Input: part model. Units: mm. Frame: model coordinates. Face numbers are marked on the shaded views. Give positions to 0.01 mm unless a question says otherwise; leave off trailing zeros. Order: outer loops, then holes, each group sorted by start corner. A loop starts at its lowest first (then second) coordinate and runs counter-clockwise, first axis right, second up.
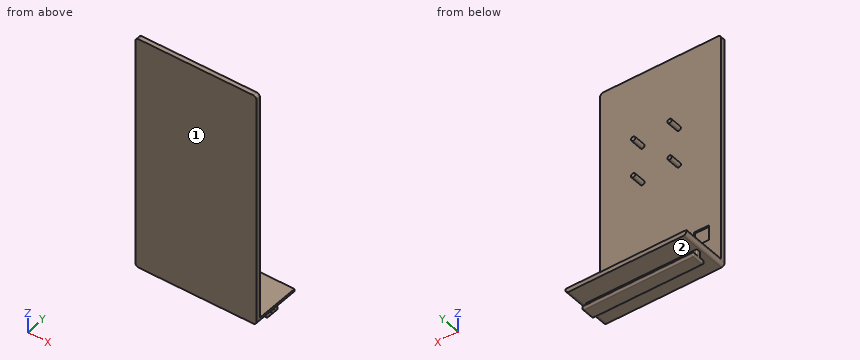
Autodesk Inventor part; units mm, degrees
ref_plane "YZ Plane" through (0, 0, 0) normal (1, 0, 0) x (0, 1, 0)
ref_plane "XZ Plane" through (0, 0, 0) normal (0, 1, 0) x (-1, 0, 0)
ref_plane "XY Plane" through (0, 0, 0) normal (0, 0, 1) x (1, 0, 0)
sketch "Sketch1" plane through (0, 0, 0) normal (0, 1, 0) x (-1, 0, 0)
  line L0 (-40, -78) -> (40, -78)
  line L1 (40, -78) -> (40, 78)
  line L2 (40, 78) -> (-40, 78)
  line L3 (-40, 78) -> (-40, -78)
  line L4 (-40, -78) -> (40, 78) construction
  line L5 (40, -78) -> (-40, 78) construction
  point P0 (0, 0)
  dimension "d0" = 80
  dimension "d1" = 156
extrude "Extrusion1" add sketch "Sketch1" along normal blind 3
sketch "Sketch2" plane through (0, 3, 0) normal (0, 1, 0) x (1, 0, 0)
  line L0 (-40, 78) -> (-40, -78)
  line L1 (-40, -78) -> (40, -78)
  line L2 (40, -78) -> (40, 78)
  line L3 (40, 78) -> (-40, 78)
  line L4 (40, 78) -> (-40, 78)
  line L5 (-40, 78) -> (-40, -78)
  line L6 (-40, -78) -> (40, -78)
  line L7 (40, -78) -> (40, 78)
  line L8 (40, 78) -> (-40, -78) construction
  line L9 (-40, 78) -> (40, -78) construction
  line L10 (37, 75) -> (-37, 75)
  line L11 (-37, 75) -> (-37, -75)
  line L12 (-37, -75) -> (37, -75)
  line L13 (37, -75) -> (37, 75)
  line L14 (37, 75) -> (-37, -75) construction
  line L15 (-37, 75) -> (37, -75) construction
  point P0 (0, 0)
  dimension "d4" = 0
  dimension "d5" = 0
  dimension "d6" = 3
  dimension "d7" = 3
extrude "Extrusion2" add sketch "Sketch2" along normal blind 30
fillet "Fillet1" radius 2 4 edges at (40, 16.5, 78) (40, 16.5, -78) (-40, 16.5, 78) (-40, 16.5, -78)
sketch "Sketch13" plane through (23.2, 5, -78) normal (0, 0, -1) x (-1, 0, 0)
  line L0 (-13.8, 18) -> (60.2, 18)
  line L1 (60.2, 18) -> (60.2, 8.4)
  line L2 (60.2, 8.4) -> (-13.8, 8.4)
  line L3 (-13.8, 8.4) -> (-13.8, 18)
  line L4 (63.2, -5) -> (63.2, 28)
  line L5 (-16.8, 28) -> (-16.8, -5)
  line L6 (-14.8, -5) -> (61.2, -5)
  point P0 (23.2, -5)
  point P1 (51.4, 0)
  point P2 (-5, 0)
  point P3 (-16.8, -5)
  point P4 (63.2, 11.5)
  point P5 (60.2, 13.2)
  dimension "d131" = 9.6
  dimension "d146" = 3
  dimension "d147" = 3
  dimension "d156" = 23
extrude "Extrusion13" add sketch "Sketch13" along normal blind 6
sketch "Sketch14" plane through (-37, 13.4, -78) normal (-1, 0, 0) x (0, 0, 1)
  line L0 (0, 9.6) -> (0, 0)
  line L1 (0, 9.6) -> (-6, 9.6)
  line L2 (-6, 0) -> (-6, 9.6)
  line L3 (0, 0) -> (-6, 0)
  line L4 (0, 9.6) -> (-3.4, 9.6)
  line L5 (-3.4, 9.6) -> (-3.4, 6.6)
  line L6 (-3.4, 6.6) -> (0, 6.6)
  line L7 (0, 6.6) -> (0, 9.6)
  line L8 (0, 0) -> (-3.4, 0)
  line L9 (-3.4, 0) -> (-3.4, 3)
  line L10 (-3.4, 3) -> (0, 3)
  line L11 (0, 3) -> (0, 0)
  point P0 (78, -13.4)
  point P1 (0, 6.6)
  dimension "d137" = 3.4
  dimension "d138" = 3
  dimension "d139" = 3.4
  dimension "d140" = 3
extrude "Extrusion14" cut sketch "Sketch14" against normal up to surface (74 mm away) contours L0 L6 L5 L1 | L0 L3 L9 L10
fillet "Fillet5" radius 1 18 edges at (0, 23, -84) (0, 23, -81.4) (0, 13.4, -84) (0, 13.4, -81.4) (-37, 16.4, -79.7) (-37, 20, -79.7) (37, 16.4, -79.7) (37, 20, -79.7) (-37, 18.2, -84) (-37, 21.5, -81.4) (-37, 14.9, -81.4) (-37, 23, -82.7) (-37, 13.4, -82.7) (37, 23, -82.7) (37, 13.4, -82.7) (37, 14.9, -81.4) (37, 18.2, -84) (37, 21.5, -81.4)
sketch "Sketch16" plane through (0, 33, 0) normal (0, 1, 0) x (1, 0, 0)
  arc A0 (-38, 78) -> (-40, 76) centre (-38, 76) ccw
  line L0 (-40, 76) -> (-40, -76)
  arc A1 (-40, -76) -> (-38, -78) centre (-38, -76) ccw
  line L1 (-38, -78) -> (38, -78)
  arc A2 (38, -78) -> (40, -76) centre (38, -76) ccw
  line L2 (40, -76) -> (40, 76)
  arc A3 (40, 76) -> (38, 78) centre (38, 76) ccw
  line L3 (38, 78) -> (-38, 78)
  line L4 (37, 75) -> (37, -75)
  line L5 (37, -75) -> (-37, -75)
  line L6 (-37, -75) -> (-37, 75)
  line L7 (-37, 75) -> (37, 75)
  line L8 (-37, 75) -> (-40, 75)
  line L9 (37, 75) -> (40, 75)
  circle A4 centre (38, 76) radius 2
  circle A5 centre (-38, 76) radius 2
  point P0 (0, 0)
  point P1 (-39.7321, 75)
  point P2 (40, 76)
  point P3 (39.7321, 75)
  dimension "d180" = 4
  dimension "d181" = 4
extrude "Extrusion16" cut sketch "Sketch16" against normal blind 30 contours L8 A5 L6 L5 L4 A4 L9 L2 A2 L1 A1 L0 | L8 L6 A5 | A4 L4 L9
sketch "Sketch18" plane through (0, 3, 0) normal (0, 1, 0) x (1, 0, 0)
  line L0 (40, 75) -> (-40, 75)
  line L1 (38, -78) -> (-38, -78)
  line L2 (40, 75) -> (40, -76)
  line L3 (32, 58) -> (22, 58)
  line L4 (22, 58) -> (22, 48)
  line L5 (22, 48) -> (32, 48)
  line L6 (32, 48) -> (32, 58)
  line L7 (-22, 48) -> (-32, 48)
  line L8 (-32, 48) -> (-32, 58)
  line L9 (-32, 58) -> (-22, 58)
  line L10 (-22, 58) -> (-22, 48)
  line L11 (38, 78) -> (-38, 78)
  line L12 (-40, -76) -> (-40, 75)
  arc A0 (-40, -76) -> (-38, -78) centre (-38, -76) ccw
  arc A1 (38, -78) -> (40, -76) centre (38, -76) ccw
  dimension "d182" = 10
  dimension "d183" = 10
  dimension "d184" = 8
  dimension "d185" = 10
  dimension "d186" = 10
  dimension "d188" = 20
  dimension "d189" = 20
extrude "Extrusion18" cut sketch "Sketch18" against normal blind 1 contours L6 L5 L4 L3 | L7 L8 L9 L10
sketch "Sketch19" plane through (0, 3, 0) normal (0, 1, 0) x (1, 0, 0)
  line L0 (40, 75) -> (40, -76)
  line L1 (38, -78) -> (-38, -78)
  line L2 (-40, -76) -> (-40, 76)
  circle A0 centre (-12.05, -3) radius 1.45
  circle A1 centre (-12.05, -28) radius 1.45
  circle A2 centre (12.05, -3) radius 1.45
  circle A3 centre (12.05, -28) radius 1.45
  line L3 (-5, -54) -> (5, -54)
  line L4 (32, 58) -> (32, 48)
  line L5 (-32, 48) -> (-32, 58)
  point P0 (40, 76)
  point P1 (0, -54)
  point P2 (0, -54)
  point P3 (32, 53)
  point P4 (-32, 53)
  dimension "d215" = 2.9
  dimension "d216" = 2.9
  dimension "d217" = 2.9
  dimension "d218" = 2.9
  dimension "d219" = 25
  dimension "d220" = 25
  dimension "d221" = 24.1
  dimension "d222" = 12.05
  dimension "d223" = 12.05
  dimension "d224" = 56
  dimension "d225" = 56
extrude "Extrusion19" add sketch "Sketch19" along normal blind 8
properties part number "module_command" material "PC/ABS Plastic"
1) Cut plane A-A (y = 5). Return the cut outline in (x, z).
2) Line query: probe 1 along Y at (x, z) = (13.5, 42.5); probe 2 along Z at (x, y) = (10.5, 9); probe 3 along Y at (x, z) = (31.5, -50). Output: solid intervals per line, ascending.
3) Cut plane C-C (z = 9.5). Return the cut outline in (x, y), then the cut area to 3 significant figures.
4) Cut plane B-B (x = -19). Return the cut outline in (y, z), then the cut area to 3 significant figures.
5) First-contact query: P1, Ø8, axis at x = -4.5, z = -51, coming from the +Y side; P2, Ø8, axis at y = 10, z = 5.5, coming from the -X side; P3, Ø8, axis at x = -17.5, y = 23, coming from the +Z side. Flat tips, straight axial feed; report the tip coordinate or a pass-through.
6) Pull-direction query (Z, two-part tool) for the marked faces 1 and 2; classes: pulls with the +Z half, pulls with the -Z half, needs draft (parallel to the pull), parting line crosses it, or undercut.
Geometry says:
1. outline: (-40, -76) arc R2 ccw to (-38, -78) - (38, -78) arc R2 ccw to (40, -76) - (40, -75) - (-40, -75) - close; circle Ø2.9 at (-12.05, 3); circle Ø2.9 at (-12.05, 28); circle Ø2.9 at (12.05, 3); circle Ø2.9 at (12.05, 28)
2. probe 1: y = 0 to 3
2. probe 2: z = -78 to -75
2. probe 3: y = 0 to 2
3. outline: (-40, 0) - (40, 0) - (40, 3) - (-40, 3) - close
3. area: 240 mm2
4. outline: (0, -78) - (16.4, -78) - (16.4, -81.4) - (14.4, -81.4) arc R1 ccw to (13.4, -82.4) - (13.4, -83) arc R1 ccw to (14.4, -84) - (22, -84) arc R1 ccw to (23, -83) - (23, -82.4) arc R1 ccw to (22, -81.4) - (20, -81.4) - (20, -78) - (33, -78) - (33, -75) - (3, -75) - (3, 78) - (0, 78) - close
4. area: 594 mm2
5. P1: stops at y = 3
5. P2: stops at x = -13.5
5. P3: stops at z = -75
6. face 1: needs draft
6. face 2: undercut
